from build123d import *

# Parameters (mm, degrees)
SKETCH_1_R      = 4
SKETCH_1_W      = 60
SKETCH_1_H      = 12
EXTRUDE_1_DEPTH = 3
EXTRUDE_START   = 35
SKETCH_2_W      = 20
SKETCH_2_H      = 20
EXTRUDE_2_DEPTH = 5
SKETCH_3_R      = 6
EXTRUDE_3_DEPTH = 6


with BuildPart() as part:
    # 草图1 → 凸台-拉伸1 (new, symmetric)
    with BuildSketch(Plane.XY):
        with BuildLine():
            Line((-35, 10), (35, 10))
            Line((35, 10), (35, -10))
            Line((35, -10), (-35, -10))
            Line((-35, -10), (-43, -10))
            ThreePointArc((-43, -10), (-53, 0), (-43, 10))
            Line((-43, 10), (-35, 10))
        make_face()
        with Locations((-43, 0)):
            Circle(SKETCH_1_R, mode=Mode.SUBTRACT)
        Rectangle(SKETCH_1_W, SKETCH_1_H, mode=Mode.SUBTRACT)
    extrude(amount=EXTRUDE_1_DEPTH, both=True)

    # 草图2 → 凸台-拉伸2 (add)
    with BuildSketch(Plane(origin=(0, 0, 0), x_dir=(0, 0, -1), z_dir=(1, 0, 0)).offset(EXTRUDE_START)):
        Rectangle(SKETCH_2_W, SKETCH_2_H)
    extrude(amount=EXTRUDE_2_DEPTH)

    # 草图3 → 凸台-拉伸3 (add, symmetric)
    with BuildSketch(Plane.XY):
        with BuildLine():
            Line((40, 10), (50, 10))
            ThreePointArc((50, 10), (60, 0), (50, -10))
            Line((50, -10), (40, -10))
            Line((40, -10), (40, 10))
        make_face()
        with Locations((50, 0)):
            Circle(SKETCH_3_R, mode=Mode.SUBTRACT)
    extrude(amount=EXTRUDE_3_DEPTH, both=True)


solid = part.part
Read the model definition and answer for the solid it produces. Units are mm, in the model's axes. A direction names the side the tool comes from. Coordinates: 2 decimals unless noted, no trailing zeros. Loops run counter-clockwise (first coordinate to the right, second up) from the corner with the lowest first, then second, coordinate; pieces in that order, holes last. Notation, with made-up numbers: (69.25, 23.5) - (80.25, 23.5) arc R19 cw to (80.25, 53.5) - close; hole circle Ø2 at (74, 56). An arc over 180 degrees is marked (long way). Answer in a Markdown table with one row per item.
Q1. The mould has two halves that part along Y. Classify faces 1 (the cylindrical face through (-53, 0, 0)), 2 (the flat face through (0, -6, 0)), 3 (the flat face through (40, 0, -8)): pulls with the +Y half, pulls with the -Y half, needs draft (parallel to the pull), parting line crosses it, or undercut.
Here are the results:
| item | result |
|---|---|
| face 1 | parting line crosses it |
| face 2 | undercut |
| face 3 | needs draft |
Q2. Find section B-B on z = 1.5. Write down the section's boundary in (x, y), plus the area to 3 significant figures.
Here are the results:
| item | result |
|---|---|
| outline | (-43, -10) - (50, -10) arc R10 ccw to (50, 10) - (-43, 10) arc R10 ccw to start; hole circle Ø8 at (-43, 0); hole (-30, -6) - (30, -6) - (30, 6) - (-30, 6) - close; hole circle Ø12 at (50, 0) |
| area | 1,290 mm^2 |
Q3. Straight lines are drawn through the part: line 1 along Y through (x, z) = (50, 3); line 2 along X through (y, z) = (0.25, 5.5); line 3 along X through (y, z) = (1, 1.5). For each, find the intervals that lie inside material, in ascending order. Write a range as [from, to].
Here are the results:
| item | result |
|---|---|
| line 1 | y = [-10, -6], [6, 10] |
| line 2 | x = [35, 44.01], [55.99, 60] |
| line 3 | x = [-52.95, -46.87], [-39.13, -30], [30, 44.08], [55.92, 59.95] |
Q4. Given P1, Ø12, axis at x = 3.5, y = -5, coming from the +Z side; P2, Ø3.5, axis at y = -3.5, z = -5.5, coming from the -X side; P3, Ø4.5, axis at y = -3, z = 7.5, coming from the +X side; P4, Ø3, axis at x = -28, y = 4, coming from the +Z side, each flat-ended and moving along its own axis, determine where each tip first touches the part or whether it passes through.
Here are the results:
| item | result |
|---|---|
| P1 | stops at z = 3 |
| P2 | stops at x = 35 |
| P3 | stops at x = 59.91 |
| P4 | passes through |
Q5. Find section D-D on y = -5. Write down the section's boundary in (x, z).
Here are the results:
| item | result |
|---|---|
| outline | (-51.66, -3) - (-30, -3) - (-30, 3) - (-51.66, 3) - close; (30, -3) - (35, -3) - (35, -10) - (40, -10) - (40, -6) - (46.68, -6) - (46.68, 6) - (40, 6) - (40, 10) - (35, 10) - (35, 3) - (30, 3) - close; (53.32, -6) - (58.66, -6) - (58.66, 6) - (53.32, 6) - close |
Q6. Find section C-C on y = 0. Write down the section's boundary in (x, z).
Here are the results:
| item | result |
|---|---|
| outline | (-53, -3) - (-47, -3) - (-47, 3) - (-53, 3) - close; (-39, -3) - (-30, -3) - (-30, 3) - (-39, 3) - close; (30, -3) - (35, -3) - (35, -10) - (40, -10) - (40, -6) - (44, -6) - (44, 6) - (40, 6) - (40, 10) - (35, 10) - (35, 3) - (30, 3) - close; (56, -6) - (60, -6) - (60, 6) - (56, 6) - close |
Q7. For faces 4 (the flat face through (43, 0, 6)), 5 (the flat face through (-8, -7, 3)), 6 (the flat face through (0, 6, 0)), 7 (the flat face through (43, 0, -6)), determine the directions among +Z, -Z, +X, -X, +Y, -Y from which every point of the face is accessible in a straight line to the end or side of a thin tool.
Here are the results:
| item | result |
|---|---|
| face 4 | +Z, +X, +Y, -Y |
| face 5 | +Z, -X, +Y, -Y |
| face 6 | +Z, -Z |
| face 7 | -Z, +X, +Y, -Y |
Q8. Find section A-A on x = 3.5. Write down the section's boundary in (y, z).
Here are the results:
| item | result |
|---|---|
| outline | (-10, -3) - (-6, -3) - (-6, 3) - (-10, 3) - close; (6, -3) - (10, -3) - (10, 3) - (6, 3) - close |
